Study the drawing (mm; zero at the part's minimum x, y, z) and answer. A direction names the side the tool comes from. Give positions to 0.01 mm unless a question says otherwise; leave off trailing zeros. Write each loop counter-clockwise with the first axis right and the second up, starting at its lowest first coordinate (ties: lowest second). Pieces come first, ordered by that corner, then holes. Notation, with made-up numbers: (3.25, 14) - (46.25, 14) arc R17 cw to (46.25, 24) - close; hole circle Ø7 at (23.25, 66). An arc over 180 degrees is marked (long way). Answer in a Markdown table with one row per item. Add a question column.
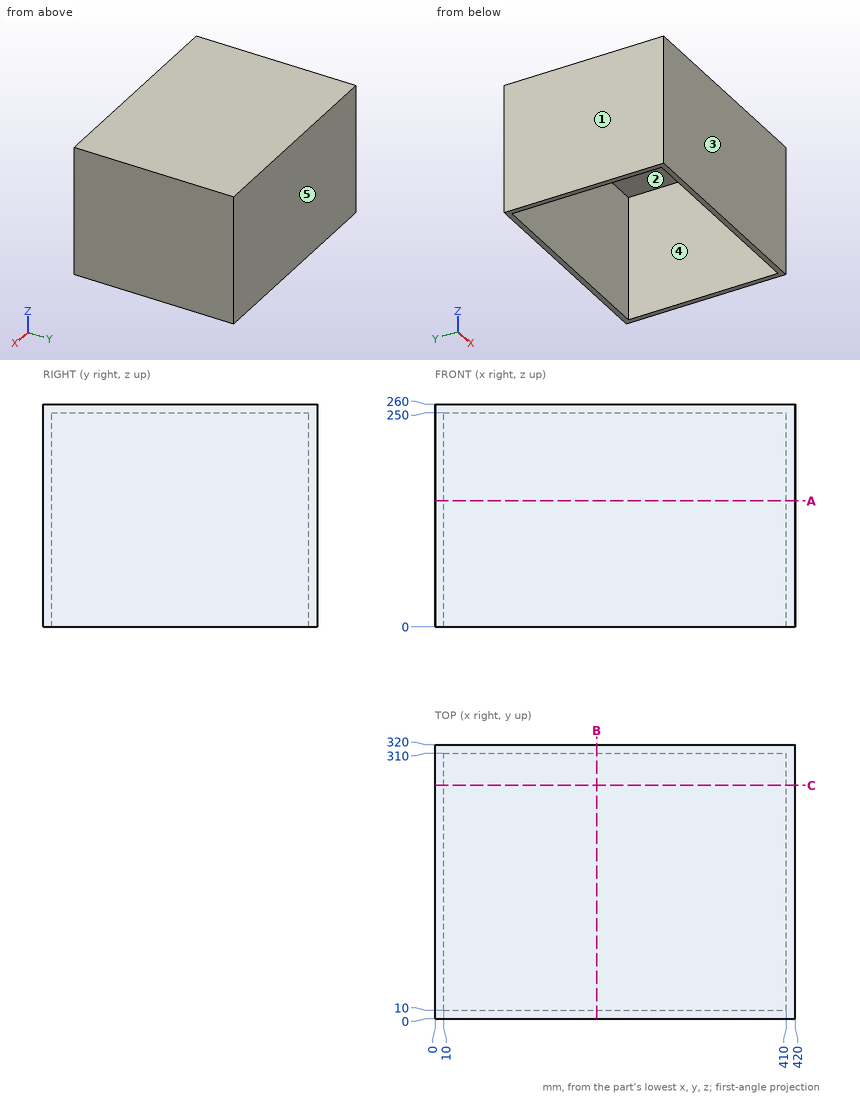
1. Given pin 1 Ø1 at (x, y) = (312, 161.5) entering from -Z; pin 2 Ø1 at (y, z) = (219.5, 109) entering from -X, each flat-ended and moving along its own axis, determine where each tip first touches the part or whether it passes through.
2. Straight lines are drawn through the part: L1, parallel to X at y = 128.5, z = 77; L2, parallel to Y at x = 243, z = 150; L3, parallel to Z at x = 316.5, y = 161. For each, find the intervals that lie inside material, in ascending order. Write a range as [from, to].
3. The mould has two halves that part along X. Classify the marked faces 1, 2 and 3: +X half, -X half, draft (parallel to the pull), parting line (faces both ways), or undercut.
4. Section C-C (y = 272.5) is taken. Give the vertices of the cut face in (x, z).
5. Section A-A (z = 147) is taken. Give the vertices of the cut face in (x, y).
6. A tool of negligible diameter and unlimited length cuts with its end or side. For the marked faces 4 and 5, from which of +Z, -Z, +X, -X, +Y, -Y can it reach the whole face along a straight path? Write none if from no direction.
7. Section B-B (x = 188.5) is taken. Give the vertices of the cut face in (y, z).
Geometry check:
| question | item | result |
|---|---|---|
| 1 | pin 1 | z = 250 |
| 1 | pin 2 | x = 0 |
| 2 | L1 | [0, 10], [410, 420] |
| 2 | L2 | [0, 10], [310, 320] |
| 2 | L3 | [250, 260] |
| 3 | face 1 | -X half |
| 3 | face 2 | undercut |
| 3 | face 3 | draft |
| 4 | outline | (0, 0) - (10, 0) - (10, 250) - (410, 250) - (410, 0) - (420, 0) - (420, 260) - (0, 260) - close |
| 5 | outline | (0, 0) - (420, 0) - (420, 320) - (0, 320) - close; hole (10, 10) - (410, 10) - (410, 310) - (10, 310) - close |
| 6 | face 4 | -Z |
| 6 | face 5 | +Z, -Z, +X, -X, +Y |
| 7 | outline | (0, 0) - (10, 0) - (10, 250) - (310, 250) - (310, 0) - (320, 0) - (320, 260) - (0, 260) - close |
